```python
from build123d import *

# Parameters (mm, degrees)
F0_W     = 10
F0_H     = 10
F1_DEPTH = 35


with BuildPart() as f1:
    # F0 (on Front) → F1 (new body, symmetric)
    with BuildSketch(Plane.XZ):
        Polygon((15, 28), (15, 38), (-15, 38), (-15, 0), (15, 0), (15, 10), (-5, 10), (-5, 28), align=None)
        with Locations((20, 5)):
            Rectangle(F0_W, F0_H)
    extrude(amount=F1_DEPTH, both=True)


solid = f1.part
```
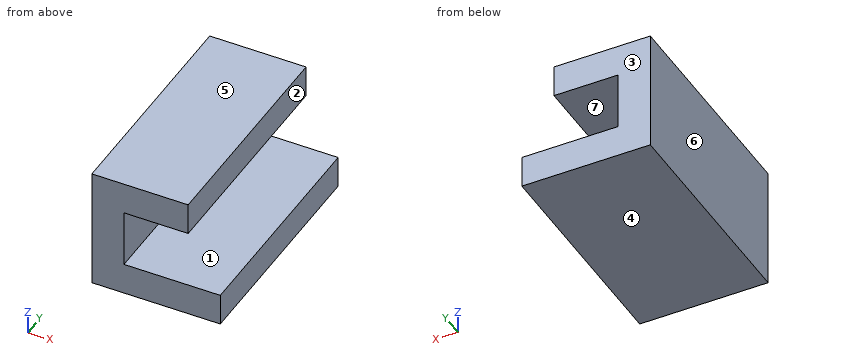
Can you work these out from the model? Positions are in its coordinate system, mm. Face numbers are marked on the shaded views. A direction names the side the tool comes from. Round coordinates to 2 decimals unless told otherwise and drop trailing zeros. Loops run counter-clockwise (first coordinate to the right, second up) from the corner with the lowest first, then second, coordinate; pieces in that order, holes last.
Item 1: Which directions (+Z, -Z, +X, -X, +Y, -Y) give clear straight access to the entire face, cutting with the end or side of a thin tool? Please do the marked faces 1, 2 and 3.
Item 2: Will these pins go through, and if not, where does the flat tip stop? pin 1 Ø8 at (x, y) = (5, 0.5) entering from -Z; pin 2 Ø3 at (y, z) = (8, 33) entering from +X; pin 3 Ø5.5 at (y, z) = (13.5, 17) entering from +X.
Item 3: Suppose I cut it at B-B, the plane y = -10.5. Write out the boundary of the cut face in (x, z), then the cut area to 3 significant figures.
Item 4: Suppose I cut it at D-D, the plane x = 20.5. Write out the boundary of the cut face in (y, z), then the cut area to 3 significant figures.
Item 5: If we mould it in two halves opening along Z, with no side actions, what happens to the marked faces 4, 5, 6 and 7? For each: +Z half, -Z half, draft (parallel to the pull), parting line (faces both ways), or undercut.
Item 6: Please list where these lines run through material, in increasing order: L1, parallel to Z at x = 8, y = -7.5; L2, parallel to X at y = 5, z = 21; L3, parallel to X at y = 6.5, z = 32.
Item 7: Suppose I cut it at C-C, the plane z = 13.5. Write out the boundary of the cut face in (x, y), then the cut area to 3 significant figures.
Item 8: Suppose I cut it at A-A, the plane x = 3. Write out the boundary of the cut face in (y, z), then the cut area to 3 significant figures.
Reported:
1. face 1: +X, +Y, -Y
1. face 2: +Z, +X, +Y, -Y
1. face 3: +Z, -Z, +X, -X, +Y
2. pin 1: stops at z = 0
2. pin 2: stops at x = 15
2. pin 3: stops at x = -5
3. outline: (-15, 0) - (25, 0) - (25, 10) - (-5, 10) - (-5, 28) - (15, 28) - (15, 38) - (-15, 38) - close
3. area: 880 mm2
4. outline: (-35, 0) - (35, 0) - (35, 10) - (-35, 10) - close
4. area: 700 mm2
5. face 4: -Z half
5. face 5: +Z half
5. face 6: draft
5. face 7: undercut
6. L1: z = 0 to 10, 28 to 38
6. L2: x = -15 to -5
6. L3: x = -15 to 15
7. outline: (-15, -35) - (-5, -35) - (-5, 35) - (-15, 35) - close
7. area: 700 mm2
8. outline: (-35, 0) - (35, 0) - (35, 10) - (-35, 10) - close; (-35, 28) - (35, 28) - (35, 38) - (-35, 38) - close
8. area: 1,400 mm2
